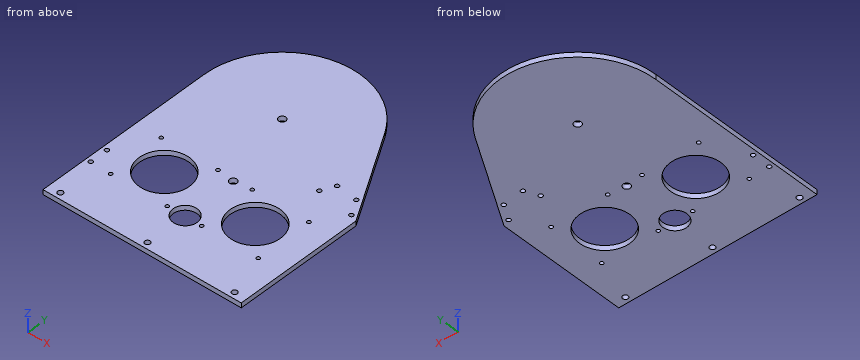
```python
from build123d import *

# Parameters (mm, degrees)
ESQUISSE1_R                     = 3
ESQUISSE1_R_2                   = 10
ESQUISSE1_R_3                   = 2.25
ESQUISSE1_R_4                   = 1.7
ESQUISSE1_R_5                   = 21
BASE_EXTRUSION_DEPTH            = 4
ESQUISSE2_R                     = 1.5
ENL_V_MAT_EXTRU_1_DEPTH         = 272.046121537
R_P_TITION_LIN_AIRE1_COUNT      = 2
R_P_TITION_LIN_AIRE1_PITCH      = 47.1
R_P_TITION_LIN_AIRE1_COUNT_DIR2 = 2
R_P_TITION_LIN_AIRE1_PITCH_DIR2 = 47.1
ESQUISSE3_R                     = 1.5
ENL_V_MAT_EXTRU_2_DEPTH         = 234.557566427
R_P_TITION_LIN_AIRE2_COUNT      = 2
R_P_TITION_LIN_AIRE2_PITCH      = 47.1
R_P_TITION_LIN_AIRE2_COUNT_DIR2 = 2
R_P_TITION_LIN_AIRE2_PITCH_DIR2 = 47.1


with BuildPart() as part:
    # Esquisse1 → Base-Extrusion (new body)
    with BuildSketch(Plane.XY):
        with BuildLine():
            Line((0, 0), (165, 0))
            Line((165, 0), (165, 106.794919243))
            Line((165, 106.794919243), (121.291651246, 182.5))
            ThreePointArc((121.291651246, 182.5), (48.176762068, 212.785178709), (0, 150))
            Line((0, 150), (0, 0))
        make_face()
        with Locations((65, 150)):
            Circle(ESQUISSE1_R, mode=Mode.SUBTRACT)
        with Locations((82.5, 40)):
            Circle(ESQUISSE1_R_2, mode=Mode.SUBTRACT)
        with Locations((82.5, 5)):
            Circle(ESQUISSE1_R_3, mode=Mode.SUBTRACT)
        with Locations((10, 5)):
            Circle(ESQUISSE1_R_3, mode=Mode.SUBTRACT)
        with Locations((155, 5)):
            Circle(ESQUISSE1_R_3, mode=Mode.SUBTRACT)
        with Locations((4, 40)):
            Circle(ESQUISSE1_R_4, mode=Mode.SUBTRACT)
        with Locations((4, 55)):
            Circle(ESQUISSE1_R_4, mode=Mode.SUBTRACT)
        with Locations((82.5, 84.807975948)):
            Circle(ESQUISSE1_R, mode=Mode.SUBTRACT)
        with Locations((44.64, 62.957975948)):
            Circle(ESQUISSE1_R_5, mode=Mode.SUBTRACT)
        with Locations((120.36, 62.957975948)):
            Circle(ESQUISSE1_R_5, mode=Mode.SUBTRACT)
        with Locations((151.537549631, 122.112567277)):
            Circle(ESQUISSE1_R_4, mode=Mode.SUBTRACT)
        with Locations((159.037549631, 109.12218622)):
            Circle(ESQUISSE1_R_4, mode=Mode.SUBTRACT)
        with Locations((128.5, 113.5)):
            Circle(ESQUISSE1_R_4, mode=Mode.SUBTRACT)
        with Locations((133.6, 124.3)):
            Circle(ESQUISSE1_R_4, mode=Mode.SUBTRACT)
    extrude(amount=BASE_EXTRUSION_DEPTH)

    # Esquisse2 → Enlèv. mat.-Extru.1 (cut, through all)
    with BuildSketch(Plane.XY.offset(4)):
        with Locations((21.09, 86.507975948)):
            Circle(ESQUISSE2_R)
    enl_v_mat_extru_1 = extrude(amount=-ENL_V_MAT_EXTRU_1_DEPTH, mode=Mode.SUBTRACT)

    # Répétition linéaire1: Enl_v. mat.-Extru.1 2 × 2
    with Locations(*[(i * R_P_TITION_LIN_AIRE1_PITCH, -j * R_P_TITION_LIN_AIRE1_PITCH_DIR2, 0) for i in range(R_P_TITION_LIN_AIRE1_COUNT) for j in range(R_P_TITION_LIN_AIRE1_COUNT_DIR2) if (i, j) != (0, 0)]):
        add(enl_v_mat_extru_1, mode=Mode.SUBTRACT)

    # Esquisse3 → Enlèv. mat.-Extru.2 (cut, through all)
    with BuildSketch(Plane(origin=(31.548888889, 23.365092485, 4), x_dir=(1, 0, 0), z_dir=(0, 0, 1))):
        with Locations((65.261111111, 63.142883463)):
            Circle(ESQUISSE3_R)
    enl_v_mat_extru_2 = extrude(amount=-ENL_V_MAT_EXTRU_2_DEPTH, mode=Mode.SUBTRACT)

    # Répétition linéaire2: Enl_v. mat.-Extru.2 2 × 2
    with Locations(*[(i * R_P_TITION_LIN_AIRE2_PITCH, -j * R_P_TITION_LIN_AIRE2_PITCH_DIR2, 0) for i in range(R_P_TITION_LIN_AIRE2_COUNT) for j in range(R_P_TITION_LIN_AIRE2_COUNT_DIR2) if (i, j) != (0, 0)]):
        add(enl_v_mat_extru_2, mode=Mode.SUBTRACT)


solid = part.part
```
Source: CAD feature listing. Evaluate the final solid. Frame: model axes, mm. Give positions to 0.01 mm unless a question says otherwise; leave off trailing zeros. Write each loop counter-clockwise with the first axis right and the second up, starting at its lowest first coordinate (ties: lowest second). Pieces come first, ordered by that corner, then holes. Notation, with made-up numbers: (-12, 45) - (39, 45) arc R8 ccw to (39, 53) - close; hole circle Ø5 at (10, -20). An arc over 180 degrees is marked (long way). One line per item, written item: value. Start each with the question number.
Q1. Section query A-A, the plane z = 2.1. Count the separate pieces of the cut face and the enclosed holes in it, then the cut area to 3 significant figures.
Q2. Section query D-D, the plane y = 170.5. Return the cut outline in (x, z).
Q3. First-contact query: pin 1 Ø1.5 at (x, z) = (59, 3) entering from +Y; pin 2 Ø5 at (x, y) = (96.81, 86.51) entering from +Z; pin 3 Ø2 at (x, z) = (28, 1.5) entering from +Y. Flat tips, straight axial feed; report the tip coordinate or a pass-through.
Q4. Material intervals for probe 1 along X at (y, z) = (64, 1); probe 2 along X at (y, z) = (148, 2.2); probe 3 along X at (y, z) = (48.5, 3.6), sorted ascending. Write a range as from..to.
Q5. Section query C-C, the plane x = 82.5. Return the cut outline in (y, z).
Q6. Section query B-B, the plane x = 44.64. Return the cut outline in (y, z), then the cut area to 3 significant figures.
Answer:
1. separate pieces: 1
1. enclosed holes: 22
1. area: 27,700 mm2
2. outline: (3.32, 0) - (128.22, 0) - (128.22, 4) - (3.32, 4) - close
3. pin 1: stops at y = 214.79
3. pin 2: stops at z = 4
3. pin 3: stops at y = 204.12
4. probe 1: x = 0..23.67, 65.61..99.39, 141.33..165
4. probe 2: x = 0..62.76, 67.24..141.21
4. probe 3: x = 0..29.41, 59.87..77.23, 87.77..105.13, 135.59..165
5. outline: (0, 0) - (2.75, 0) - (2.75, 4) - (0, 4) - close; (7.25, 0) - (30, 0) - (30, 4) - (7.25, 4) - close; (50, 0) - (81.81, 0) - (81.81, 4) - (50, 4) - close; (87.81, 0) - (212.6, 0) - (212.6, 4) - (87.81, 4) - close
6. outline: (0, 0) - (41.96, 0) - (41.96, 4) - (0, 4) - close; (83.96, 0) - (211.73, 0) - (211.73, 4) - (83.96, 4) - close
6. area: 679 mm2
